Autodesk Inventor part; units mm, degrees
ref_plane "YZ Plane" through (0, 0, 0) normal (1, 0, 0) x (0, 1, 0)
ref_plane "XZ Plane" through (0, 0, 0) normal (0, 1, 0) x (-1, 0, 0)
ref_plane "XY Plane" through (0, 0, 0) normal (0, 0, 1) x (1, 0, 0)
sketch "Sketch1" plane through (0, 0, 0) normal (0, 0, 1) x (1, 0, 0)
  line L0 (-17.78, 0) -> (17.78, 0)
  line L1 (0, -17.78) -> (0, 17.78)
  line L2 (-12.7, 12.7) -> (12.7, 12.7)
  line L3 (12.7, 12.7) -> (12.7, -12.7)
  line L4 (12.7, -12.7) -> (-12.7, -12.7)
  line L5 (-12.7, -12.7) -> (-12.7, 12.7)
  line L6 (9.525, 9.525) -> (-9.525, 9.525)
  line L7 (-9.525, 9.525) -> (-9.525, -9.525)
  line L8 (-9.525, -9.525) -> (9.525, -9.525)
  line L9 (9.525, -9.525) -> (9.525, 9.525)
  point P0 (0, 0)
  point P1 (-12.7, 0)
  point P2 (0, 12.7)
  dimension "d0" = 25.4
  dimension "d1" = 3.175
extrude "Extrusion1" add sketch "Sketch1" along normal mid plane 381 contours L5 L2 L1 L6 L7 L0 | L0 L7 L8 L1 L4 L5 | L1 L8 L9 L0 L3 L4 | L2 L3 L0 L9 L6 L1
sketch "Sketch3" plane through (-12.7, 12.7, 190.5) normal (0, 1, 0) x (1, 0, 0)
  line L0 (0, 0) -> (25.4, 0)
  line L1 (25.4, 0) -> (25.4, 381)
  line L2 (0, 0) -> (25.4, 14.6647)
  point P0 (12.7, 190.5)
  dimension "d7" = 30
extrude "Extrusion3" cut sketch "Sketch3" against normal through all
properties part number "tubing_template_0.125" material "Aluminum-6061"
Input: part model. Units: mm. Frame: model coordinates. A direction names the side the tool comes from. Coordinates: 2 decimals unless noted, no trailing zeros. Loops run counter-clockwise (first coordinate to the right, second up) from the corner with the lowest first, then second, coordinate; pieces in that order, holes last. Notation, with made-up numbers: (28, -1) -> (54, -1) arc R8 cw to (54, 8) -> close; hole circle Ø1 at (-27.5, 18). An arc over 180 degrees is marked (long way). Write item = value, one per line. Start each with the question number.
Item 1: Cut plane C-C, the plane x = 1.5. Return loops of the section in (y, z) (3 decimals).
Item 2: Cut plane B-B, the plane z = -11. Return loops of the section in (x, y) (3 decimals), plus the area to 3 significant figures.
Item 3: Material intervals for line 1 (Y direction, x = -2.25, z = -86) (3 decimals); line 2 (Z direction, x = 11, y = -8.25), sorted ascending.
Item 4: Reachability of faces 1 (the face through (0, -12.7, -3)), 2 (the face through (9.525, 0, -9)) from +Z, -Z, +X, -X, +Y, -Y: full face, straight path, thin tool, end or side. Return the list, or none.
Item 5: Cut plane A-A, the plane y = 5.5. Return loops of the section in (x, z) (3 decimals).
Item 6: Mould query, pull axis Y, two halves, no side actions, for faces 3 (the face through (12.7, 0, -10)), 4 (the face through (0, 12.7, -3)), 5 (the face through (-9.525, 0, -4)). Classes: pulls with the +Y half, pulls with the -Y half, needs draft (parallel to the pull), parting line crosses it, or undercut.
Ans:
q1.outline = (-12.7, -190.5) -> (-9.525, -190.5) -> (-9.525, 182.302) -> (-12.7, 182.302) -> close; (9.525, -190.5) -> (12.7, -190.5) -> (12.7, 182.302) -> (9.525, 182.302) -> close
q2.outline = (-12.7, -12.7) -> (12.7, -12.7) -> (12.7, 12.7) -> (-12.7, 12.7) -> close; hole (-9.525, -9.525) -> (9.525, -9.525) -> (9.525, 9.525) -> (-9.525, 9.525) -> close
q2.area = 282 mm²
q3.line_1 = -12.7 to -9.525, 9.525 to 12.7
q3.line_2 = -190.5 to 176.82
q4.face_1 = +Z, -Z, +X, -X, -Y
q4.face_2 = +Z, -Z
q5.outline = (-12.7, -190.5) -> (-9.525, -190.5) -> (-9.525, 188.667) -> (-12.7, 190.5) -> close; (9.525, -190.5) -> (12.7, -190.5) -> (12.7, 175.835) -> (9.525, 177.668) -> close
q6.face_3 = needs draft
q6.face_4 = pulls with the +Y half
q6.face_5 = undercut
